Input: part model. Units: mm. Frame: model coordinates. Coordinates: 2 decimals unless noted, no trailing zeros. Write each loop counter-clockwise with the first axis right and the second up, starting at its lowest first coordinate (ties: lowest second). Pieces come first, ordered by that corner, then holes.
from build123d import *

# Parameters (mm, degrees)
BOSS_EXTRUDE1_DEPTH = 1
SKETCH2_R           = 1.1
CUT_EXTRUDE1_DEPTH  = 4
FILLET1_R           = 2


with BuildPart() as part:
    # Sketch1 → Boss-Extrude1 (new body)
    with BuildSketch(Plane(origin=(0, 0, 0), x_dir=(1, 0, 0), z_dir=(0, 1, 0))):
        Polygon((52, 77), (52, 87), (0, 87), (0, 0), (52, 0), (52, 57), (72, 57), (72, 77), align=None)
    extrude(amount=BOSS_EXTRUDE1_DEPTH)

    # Sketch2 → Cut-Extrude1 (cut)
    with BuildSketch(Plane(origin=(0, 1, 0), x_dir=(1, 0, 0), z_dir=(0, 1, 0))):
        with Locations((4, 2)):
            Circle(SKETCH2_R)
        with Locations((48, 2)):
            Circle(SKETCH2_R)
        with Locations((24, 85)):
            Circle(SKETCH2_R)
        with Locations((50, 75)):
            Circle(SKETCH2_R)
    extrude(amount=-CUT_EXTRUDE1_DEPTH, mode=Mode.SUBTRACT)

    # Fillet1
    fillet1_edges = [part.edges().sort_by_distance(p)[0] for p in [
        (0, 0.5, -87),
        (52, 0.5, -87),
        (52, 0.5, -77),
        (72, 0.5, -77),
        (72, 0.5, -57),
        (52, 0.5, -57),
        (52, 0.5, 0),
        (0, 0.5, 0),
    ]]
    fillet(fillet1_edges, radius=FILLET1_R)


solid = part.part
Item 1: Section query D-D, the plane z = -10. Return loops of the section in (x, y), then the cut area to 3 significant figures.
Item 2: Pin query (flat end, axial travel): pin 1 Ø3 at (x, z) = (48, -2) entering from -Y; pin 2 Ø0.5 at (y, z) = (0.5, -40) entering from +X. Return the tip coordinate at first contact, or that it passes through.
Item 3: Pull-direction query (Z, two-part tool) for faces 1 (the face through (49.189, 0.507, -75.743)), 2 (the face through (49.05, 0.51, -2.33)), 3 (the face through (0.57, 0.51, -0.6)), 4 (the face through (27, 0, -44)); classes: released by +Z, released by -Z, zero draft, split by the parting line, or undercut.
Item 4: Section query A-A, the plane x = 24. Return loops of the section in (y, z).
Item 5: Section query B-B, the plane y = 0.8. Return loops of the section in (x, z), then the cut area to 3 significant figures.
Item 6: Material intervals for line 1 (X direction, y = 0.65, z = -85); line 2 (Z direction, x = 50, y = 0.3); line 3 (Z direction, x = 4, y = 0.2), sorted ascending.
Item 7: Section query C-C, the plane x = 64.5. Return loops of the section in (y, z), then the cut area to 3 significant figures.
The answers:
1. outline: (0, 0) - (52, 0) - (52, 1) - (0, 1) - close
1. area: 52.0 mm2
2. pin 1: stops at y = 0
2. pin 2: stops at x = 52
3. face 1: undercut
3. face 2: undercut
3. face 3: released by +Z
3. face 4: zero draft
4. outline: (0, -87) - (1, -87) - (1, -86.1) - (0, -86.1) - close; (0, -83.9) - (1, -83.9) - (1, 0) - (0, 0) - close
5. outline: (0, -85) arc R2 ccw to (2, -87) - (50, -87) arc R2 ccw to (52, -85) - (52, -79) arc R2 cw to (54, -77) - (70, -77) arc R2 ccw to (72, -75) - (72, -59) arc R2 ccw to (70, -57) - (54, -57) arc R2 cw to (52, -55) - (52, -2) arc R2 ccw to (50, 0) - (2, 0) arc R2 ccw to (0, -2) - close; hole circle Ø2.2 at (4, -2); hole circle Ø2.2 at (24, -85); hole circle Ø2.2 at (48, -2); hole circle Ø2.2 at (50, -75)
5. area: 4,910 mm2
6. line 1: x = 0 to 22.9, 25.1 to 52
6. line 2: z = -87 to -76.1, -73.9 to 0
6. line 3: z = -87 to -3.1, -0.9 to 0
7. outline: (0, -77) - (1, -77) - (1, -57) - (0, -57) - close
7. area: 20.0 mm2
